Verification items for the finished model (mm, model axes). A direction names the side the tool comes from. Round coordinates to 2 decimals unless told otherwise and drop trailing zeros. Loops run counter-clockwise (first coordinate to the right, second up) from the corner with the lowest first, then second, coordinate; pieces in that order, holes last. Notation, with made-up numbers: (66.25, 25.5) -> (122.25, 25.5) arc R22 ccw to (122.25, 45.5) -> close; hole circle Ø4 at (-40, 76.5). An arc over 180 degrees is marked (long way). Write item = value, one per line.
Autodesk Inventor part; units mm, degrees
ref_plane "Work Plane2" through (48.1, 0, 0) normal (1, 0, 0) x (0, 0, -1)
ref_plane "Work Plane3" through (0, 10, 0) normal (0, 1, 0) x (-1, 0, 0)
ref_plane "Work Plane4" through (20.15, 0, 0) normal (1, 0, 0) x (0, 1, 0)
sketch "Sketch1" plane through (0, 0, 0) normal (0, 0, 1) x (1, 0, 0)
  line L0 (0, 0) -> (40.3, 0)
  line L1 (40.3, 0) -> (40.3, 20)
  line L2 (40.3, 20) -> (0, 20)
  line L3 (0, 20) -> (0, 0)
  dimension "d0" = 40.3
  dimension "d1" = 20
extrude "Extrusion1" add sketch "Sketch1" along normal blind 37
sketch "Sketch2" plane through (40.3, 0, 0) normal (1, 0, 0) x (0, 0, -1)
  line L0 (0, 20) -> (-37, 20)
  line L1 (-37, 0) -> (-37, 20)
  line L2 (0, 0) -> (-37, 0)
  line L3 (-31.5, 0) -> (-28.2, 0)
  line L4 (-28.2, 0) -> (-28.2, 20)
  line L5 (-28.2, 20) -> (-31.5, 20)
  line L6 (-31.5, 20) -> (-31.5, 0)
  dimension "d4" = 3.3
  dimension "d5" = 5.5
extrude "Extrusion2" add sketch "Sketch2" along normal blind 6.8 contours L4 L2 L6 L0
sketch "Sketch3" plane through (40.3, 0, 31.5) normal (0, 0, 1) x (1, 0, 0)
  line L0 (6.8, 20) -> (6.8, 0)
  line L1 (0, 20) -> (6.8, 20)
  circle A0 centre (4, 15.7) radius 2.2
  point P0 (-40.3, 0)
  dimension "d8" = 4.4
  dimension "d9" = 2.8
  dimension "d10" = 4.3
extrude "Extrusion3" cut sketch "Sketch3" against normal through all
ref_plane "Work Plane2" through (48.1, 0, 0) normal (1, 0, 0) x (0, 0, -1)
sketch "Sketch7" plane through (48.1, 0, 0) normal (1, 0, 0) x (0, 0, -1)
  line L0 (-31.5, 16.9) -> (-28.2, 16.9)
  line L1 (-28.2, 14.5) -> (-31.5, 14.5)
  line L2 (-31.5, 16.9) -> (-28.2, 16.9)
  line L3 (-28.2, 16.9) -> (-28.2, 14.5)
  line L4 (-28.2, 14.5) -> (-31.5, 14.5)
  line L5 (-31.5, 14.5) -> (-31.5, 16.9)
  point P0 (0, 0)
extrude "Extrusion5" cut sketch "Sketch7" against normal blind 3
ref_plane "Work Plane3" through (0, 10, 0) normal (0, 1, 0) x (-1, 0, 0)
mirror "Mirror1" about plane through (0, 10, 0) normal (0, 1, 0) of "Extrusion3", "Extrusion5"
ref_plane "Work Plane4" through (20.15, 0, 0) normal (1, 0, 0) x (0, 1, 0)
mirror "Mirror2" about plane through (20.15, 0, 0) normal (1, 0, 0) of "Extrusion2", "Extrusion3", "Extrusion5", "Mirror1"
sketch "Sketch8" plane through (0, 0, 37) normal (0, 0, 1) x (1, 0, 0)
  line L0 (40.3, 0) -> (40.3, 20)
  line L1 (40.3, 20) -> (0, 20)
  line L2 (0, 20) -> (0, 0)
  line L3 (34.6, 18.9) -> (14.5596, 18.9)
  line L4 (14.5596, 1.1) -> (34.6, 1.1)
  arc A0 (14.5596, 18.9) -> (14.5596, 1.1) centre (10, 10) ccw
  arc A1 (34.6, 6.0336) -> (34.6, 13.9664) centre (30.3, 10) ccw
  line L5 (34.6, 1.1) -> (34.6, 6.0336)
  line L6 (34.6, 13.9664) -> (34.6, 18.9)
  dimension "d27" = 1.1
  dimension "d29" = 20
  dimension "d30" = 10
  dimension "d31" = 11.7
  dimension "d32" = 10
extrude "Extrusion6" add sketch "Sketch8" along normal blind 2 contours A0 L3 L6 A1 L5 L4
sketch "Sketch9" plane through (0, 0, 39) normal (0, 0, 1) x (1, 0, 0)
  arc A0 (14.5596, 18.9) -> (14.5596, 1.1) centre (10, 10) ccw
  circle A1 centre (10, 10) radius 6.5
  point P0 (0, 0)
  dimension "d35" = 13
extrude "Extrusion7" add sketch "Sketch9" along normal blind 1.7
sketch "Sketch10" plane through (10, 10, 40.7) normal (0, 0, 1) x (1, 0, 0)
  circle A0 centre (0, 0) radius 6.5
  circle A1 centre (0, 0) radius 5.55
  point P0 (-10, -10)
  dimension "d38" = 11.1
extrude "Extrusion8" add sketch "Sketch10" along normal blind 0.4 contours A1
sketch "Sketch11" plane through (10, 10, 41.1) normal (0, 0, 1) x (1, 0, 0)
  circle A0 centre (0, 0) radius 5.55
  circle A1 centre (0, 0) radius 2.95
  point P0 (-10, -10)
  dimension "d41" = 5.9
extrude "Extrusion9" add sketch "Sketch11" along normal blind 4 contours A1
ref_plane "ConstraintPlane" through (10, 0, 0) normal (1, 0, 0) x (0, 1, 0)
properties part number "MG996RServo"
(1) Sectioned sample at D-D, the plane z = 42. Record the cut outline in (x, y).
Filled sheet:
outline = circle Ø5.9 at (10, 10)
(2) Set-up check for faces 1 (the face through (2, 2, 37)), 2 (the face through (40.3, 10, 14)), 3 (the face through (0, 10, 34)), 4 (the face through (7.053, 9.87, 43.072)), 5 (the face through (24, 1.1, 38)): record each of +Z, -Z, +X, -X, +Y, -Y from which the full face is reachable in a straight line by a thin tool's end or side.
Filled sheet:
face_1 = +Z, -X, -Y
face_2 = -Z, +X, +Y, -Y
face_3 = +Z, -X, +Y, -Y
face_4 = +Z
face_5 = +Z, +X, -Y
(3) Sectioned sample at C-C, the plane z = 14. Record the cut outline in (x, y), and give its area (3 significant figures).
Filled sheet:
outline = (0, 0) -> (40.3, 0) -> (40.3, 20) -> (0, 20) -> close
area = 806 mm2
(4) Go/stop test with flat-tipped pins: pin 1 Ø4 at (x, y) = (44.3, 4.3) entering from +Z; pin 2 Ø3 at (x, y) = (3, 6.5) entering from +Z; pin 3 Ø6 at (x, y) = (0.5, 6.5) entering from +Z; pin 4 Ø4 at (y, z) = (6, 16) entering from +X. Record where each tip stops, or that it passes through.
Filled sheet:
pin_1 = through
pin_2 = 40.7
pin_3 = 39
pin_4 = 40.3
(5) Draft check along Y on faces 6 (the face through (12.4, 7.6, 41.1)), 7 (the face through (42.1, 15.78, 29.87)), 8 (the face through (25, 18.9, 38)). Enter one of: released by +Y, released by -Y, zero draft, split by the parting line, or undercut.
Filled sheet:
face_6 = zero draft
face_7 = undercut
face_8 = released by +Y
(6) Material ranges on probe 1 along Y at (x, z) = (-4, 29.5); probe 2 along X at (y, z) = (2.75, 29); probe 3 along Z at (x, y) = (36, 10.5), recorded low to high. Write a range as from..to.
Filled sheet:
probe_1 = 0..2.1, 6.5..13.5, 17.9..20
probe_2 = -6.8..-5.56, -2.44..42.74, 45.86..47.1
probe_3 = 0..39
(7) Sectioned sample at A-A, the plane x = -4. Record the cut outline in (y, z), and give its area (3 significant figures).
Filled sheet:
outline = (0, 28.2) -> (2.1, 28.2) -> (2.1, 31.5) -> (0, 31.5) -> close; (6.5, 28.2) -> (13.5, 28.2) -> (13.5, 31.5) -> (6.5, 31.5) -> close; (17.9, 28.2) -> (20, 28.2) -> (20, 31.5) -> (17.9, 31.5) -> close
area = 37.0 mm2
(8) Sectioned sample at B-B, the plane x = 25.5. Record the cut outline in (y, z), and give its area (3 significant figures).
Filled sheet:
outline = (0, 0) -> (20, 0) -> (20, 37) -> (18.9, 37) -> (18.9, 39) -> (1.1, 39) -> (1.1, 37) -> (0, 37) -> close
area = 776 mm2
